from build123d import *

# Parameters (mm, degrees)
PAD118_DEPTH            = 90
POCKET084_DEPTH         = 90.001
SKETCH238_R             = 2
POCKET085_DEPTH         = 10
POCKET085_TAPER         = 5
SKETCH239_W             = 5.7
SKETCH239_H             = 15
PAD119_DEPTH            = 4
BODY139_ROLL_ANGLE      = 90
BODY139_PLACEMENT_ANGLE = 180


with BuildPart() as part:
    # Sketch236 (on Face1 of CopyLinearPattern013) → Pad118 (new body)
    with BuildSketch(Plane(origin=(0, 240, 0), x_dir=(-1, 0, 0), z_dir=(0, 1, 0))):
        Polygon((10, 3.1), (10, -3.1), (8, -3.1), (8, -5.5), (6.3, -5.5), (3.9, -3.1), (3.9, 3.1), (6.3, 5.5), (8, 5.5), (8, 3.1), align=None)
    extrude(amount=PAD118_DEPTH)

    # Sketch237 (on Face11 of Pad118) → Pocket084 (cut, through all)
    with BuildSketch(Plane.XZ.offset(-240)):
        Polygon((-8, 5.1), (-8, 5.5), (-6.3, 5.5), (-3.9, 3.1), (-3.9, -3.1), (-6.3, -5.5), (-8, -5.5), (-8, -5.1), (-6.465685, -5.1), (-4.3, -2.934315), (-4.3, 2.934315), (-6.465685, 5.1), align=None)
    extrude(amount=-POCKET084_DEPTH, mode=Mode.SUBTRACT)

    # Sketch238 (on Face1 of Pocket084) → Pocket085 (cut)
    with BuildSketch(Plane(origin=(-10, 0, 0), x_dir=(0, -1, 0), z_dir=(-1, 0, 0))):
        with Locations((-310, 0)):
            Circle(SKETCH238_R)
        with Locations((-302, 0)):
            Circle(SKETCH238_R)
        with Locations((-318, 0)):
            Circle(SKETCH238_R)
    extrude(amount=-POCKET085_DEPTH, taper=POCKET085_TAPER, mode=Mode.SUBTRACT)

    # Sketch239 (on Face3 of Pocket085) → Pad119 (join)
    with BuildSketch(Plane.XZ.offset(-240)):
        with Locations((-7.15, 0)):
            Rectangle(SKETCH239_W, SKETCH239_H)
    extrude(amount=PAD119_DEPTH)


with BuildPart() as part_1:
    # Body139 roll: moved
    add(part.part.rotate(Axis((0, 0, 0), (1, 0, 0)), BODY139_ROLL_ANGLE))


with BuildPart() as part_2:
    # Body139 placement: moved
    add(part_1.part.moved(Location((-41, 229.5, -133))).rotate(Axis((-41, 229.5, -133), (0, 0, 1)), BODY139_PLACEMENT_ANGLE))


solid = part_2.part
For this review, take the finished solid that the model builds, in its own axes (mm). A direction names the side the tool comes from. Round coordinates to 2 decimals unless told otherwise and drop trailing zeros. Order: outer loops, then holes, each group sorted by start corner. A loop starts at its lowest first (then second) coordinate and runs counter-clockwise, first axis right, second up. Notation, with made-up numbers: (32.25, 48) -> (50.25, 48) arc R13 cw to (50.25, 52) -> close; hole circle Ø5 at (-4.75, 68). An arc over 180 degrees is marked (long way). Write item = value, one per line. Start each with the question number.
1) The part is to be moulded in two halves that separate along Y. For faces 1 (the face through (-34, 234.6, 151)), 2 (the face through (-34, 230, 103)), 3 (the face through (-33.89, 229.577, 186.745)), say which applies: +Y half, -Y half, draft (parallel to the pull), parting line (faces both ways), or undercut.
2) Take a section at B-B on z = 137. State the section outline as (x, y) points.
3) Take a section at D-D on z = 169. State the section outline as (x, y) points, plus the area to 3 significant figures.
4) Take a section at C-C on y = 233.5. State the section outline as (x, z) points, plus the area to 3 significant figures.
5) To check wall thickness, follow line 1 (Z direction, x = -32.35, y = 228.5); line 2 (Z direction, x = -33.05, y = 231); line 3 (Y direction, x = -32.7, z = 151). State the ranges of each line that lie inside material, in increasing order. Write a range as from..to.
6) Tool access review of faces 4 (the face through (-35.602, 225.468, 151.37)), 5 (the face through (-32, 226.4, 151)), 6 (the face through (-35.632, 233.502, 151.37)): name each direction out of +Z, -Z, +X, -X, +Y, -Y from which nothing blocks a thin tool from reaching the whole face with its end or side.
7) Insertion check: pin 1 (0.5 mm diameter, centred on x = -34, z = 172.5, fed in from +Y); pin 2 (1 mm diameter, centred on y = 234, z = 161, fed in from +X); pin 3 (3 mm diameter, centred on x = -35, z = 129.5, fed in from -Y). Each pin has a flat end and moves straight along its axis. Give the tip position at first contact, or say it passes through.
8) Take a section at A-A on x = -31.8. State the section outline as (y, z) points, plus the area to 3 significant figures.
Verdict:
q1.face_1 = +Y half
q1.face_2 = draft
q1.face_3 = undercut
q2.outline = (-36.7, 226.57) -> (-34.53, 224.4) -> (-33, 224.4) -> (-33, 226.4) -> (-31, 226.4) -> (-31, 232.6) -> (-33, 232.6) -> (-33, 234.6) -> (-34.53, 234.6) -> (-36.7, 232.43) -> close
q3.outline = (-36.7, 226.57) -> (-34.53, 224.4) -> (-33, 224.4) -> (-33, 226.4) -> (-31, 226.4) -> (-31, 227.5) -> (-36.7, 228) -> close; (-36.7, 231) -> (-31, 231.5) -> (-31, 232.6) -> (-33, 232.6) -> (-33, 234.6) -> (-34.53, 234.6) -> (-36.7, 232.43) -> close
q3.area = 25.5 mm2
q4.outline = (-36.7, 103) -> (-31, 103) -> (-31, 107) -> (-33, 107) -> (-33, 197) -> (-35.63, 197) -> (-35.63, 107) -> (-36.7, 107) -> close
q4.area = 260 mm2
q5.line_1 = 103..167.41, 170.59..175.41, 178.59..183.41, 186.59..197
q5.line_2 = 103..167.97, 170.03..175.97, 178.03..183.97, 186.03..197
q5.line_3 = 226.4..232.6
q6.face_4 = +Z, -X, -Y
q6.face_5 = +Z, +X, -Y
q6.face_6 = +Z, -X, +Y
q7.pin_1 = 234.6
q7.pin_2 = -33
q7.pin_3 = 224.4
q8.outline = (222, 103) -> (237, 103) -> (237, 107) -> (232.6, 107) -> (232.6, 197) -> (226.4, 197) -> (226.4, 107) -> (222, 107) -> close; hole circle Ø3.86 at (229.5, 169); hole circle Ø3.86 at (229.5, 177); hole circle Ø3.86 at (229.5, 185)
q8.area = 583 mm2
